The listing builds one solid part. Answer for the finished solid, in the listing's coordinates (mm). Face numbers are marked on the shaded views. A direction names the side the tool comes from. Coordinates: 2 decimals unless noted, no trailing zeros. Order: outer loops, then holes, each group sorted by start corner. A loop starts at its lowest first (then second) coordinate and runs counter-clockwise, first axis right, second up.
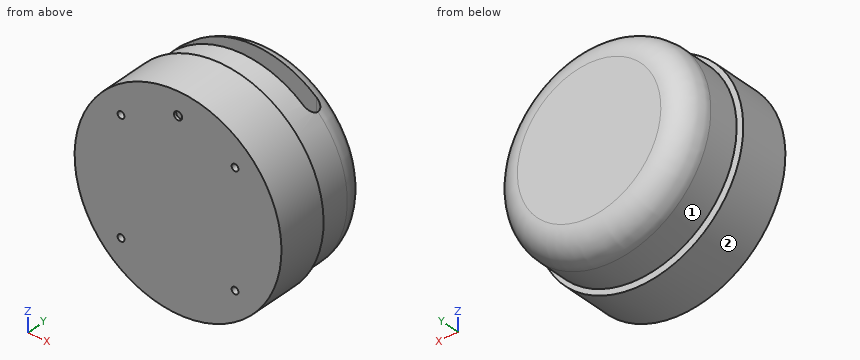
from build123d import *

# Parameters (mm, degrees)
SKETCH_2_R               = 1.5
CUT_EXTRUDE_1_DEPTH      = 1
PATTERN_CIRCULAR_1_COUNT = 4
FILLET_1_R               = 10
CUT_EXTRUDE_2_DEPTH      = 68.420234722


with BuildPart() as part:
    # 草图1 → 旋转1 (revolve)
    with BuildSketch(Plane.XY, mode=Mode.PRIVATE) as revolve_1_sk:
        Polygon((0, 0), (-37.845, 0), (-37.845, 18.6), (-34, 18.6), (-34, 19.6), (-36.25, 19.6), (-36.25, 41), (0, 41), align=None)
    revolve(revolve_1_sk.sketch.rotate(Axis((0, 49.444830204, 0), (0, -1, 0)), 270), axis=Axis((0, 49.444830204, 0), (0, -1, 0)))

    # 草图2 → 切除-拉伸1 (cut)
    with BuildSketch(Plane.XZ):
        with Locations(Location((0, 29.5, 0), (0, 0, 270))):
            Circle(SKETCH_2_R)
    extrude(amount=-CUT_EXTRUDE_1_DEPTH, mode=Mode.SUBTRACT)

    # 草图4 → g (revolve, cut)
    with BuildSketch(Plane(origin=(-20.859650045, 0, 20.859650045), x_dir=(0, 0, -1), z_dir=(1, 0, 0))):
        Polygon((0, 0), (0, 8.251075774), (1.25, 7.5), (1.25, 0), align=None)
    hole_wizard_g = revolve(axis=Axis((-20.859650045, -6.35, 20.859650045), (0, 1, 0)), mode=Mode.SUBTRACT)

    # 阵列(圆周)1: g ×4 about axis
    pattern_circular_1_axis = Axis((0, 0, 0), (0, 1, 0))
    for i in range(1, PATTERN_CIRCULAR_1_COUNT):
        add(hole_wizard_g.rotate(pattern_circular_1_axis, i * 360 / PATTERN_CIRCULAR_1_COUNT), mode=Mode.SUBTRACT)

    # 圆角1
    fillet_1_edges = [part.edges().sort_by_distance(p)[0] for p in [
        (0, 41, -36.25),
    ]]
    fillet(fillet_1_edges, radius=FILLET_1_R)

    # 草图5 → 切除-拉伸2 (cut, through all)
    with BuildSketch(Plane.XY):
        with BuildLine():
            Line((-22.5, 34), (22.5, 34))
            ThreePointArc((22.5, 34), (25.5, 31), (22.5, 28))
            Line((22.5, 28), (-22.5, 28))
            ThreePointArc((-22.5, 28), (-25.5, 31), (-22.5, 34))
        make_face()
    extrude(amount=CUT_EXTRUDE_2_DEPTH, mode=Mode.SUBTRACT)


solid = part.part
(1) Find section A-A on y = 5.5. Determine the outline of the cut face in (x, z) (3 decimals).
(2) Find the intervals of material crossed by probe 1 along Y at (x, z) = (-12, 34); probe 2 along Y at (x, z) = (-8.5, 16); probe 3 along Y at (x, z) = (17.5, 30), in increasing order.
(3) A tool of negligible diameter and unlimited length cuts with its end or side. For the marked faces 1 and 2, from which of +Z, -Z, +X, -X, +Y, -Y can it reach the whole face along a straight path? Write none if from no direction.
(4) Given pin 1 Ø2 at (x, z) = (-20.86, -20.86) entering from -Y; pin 2 Ø1.5 at (x, y) = (-5, 16.5) entering from -Z; pin 3 Ø1 at (x, y) = (21.5, 17) entering from -Z, each flat-ended and moving along its own axis, determine where each tip first touches the part or whether it passes through.
(5) Find section B-B on y = 10. Determine the outline of the cut face in (x, z) (3 decimals).
Resolved:
1. outline: circle Ø75.69 at (0, 0); hole circle Ø2.5 at (-20.86, -20.86); hole circle Ø2.5 at (-20.86, 20.86); hole circle Ø2.5 at (20.86, -20.86); hole circle Ø2.5 at (20.86, 20.86)
2. probe 1: y = 0 to 18.6, 19.6 to 28
2. probe 2: y = 0 to 28, 34 to 41
2. probe 3: y = 0 to 18.6, 19.6 to 28, 34 to 36.3
3. face 1: +Y
3. face 2: +Y, -Y
4. pin 1: stops at y = 7.65
4. pin 2: stops at z = -37.61
4. pin 3: stops at z = -31.48
5. outline: circle Ø75.69 at (0, 0)
